Model file for the job. Use its own axes, mm. A direction names the side the tool comes from. Give positions to 0.01 mm unless a question says otherwise; leave off trailing zeros. Write each loop counter-clockwise with the first axis right and the second up, starting at its lowest first coordinate (ties: lowest second). Pieces come first, ordered by that corner, then holes. Notation, with made-up numbers: (-36, 25) - (1, 25) arc R38 cw to (1, 64) - close; hole circle Ø1 at (-24, -14.75). An arc over 180 degrees is marked (long way). Use a Markdown table: item, result. Add a question column.
```python
from build123d import *

# Parameters (mm, degrees)
BOSS_EXTRUDE1_DEPTH = 20
SKETCH8_W           = 42
SKETCH8_H           = 60
CUT_EXTRUDE1_DEPTH  = 15
CUT_EXTRUDE2_START  = -5
CUT_EXTRUDE2_DEPTH  = 5
SKETCH10_R          = 36
CUT_EXTRUDE3_DEPTH  = 159.144630057
SKETCH11_R          = 41
SKETCH11_R_2        = 36
BOSS_EXTRUDE4_DEPTH = 5
SKETCH2_W           = 108.205781707
SKETCH2_H           = 80
SKETCH2_R           = 3
BOSS_EXTRUDE6_DEPTH = 20


# Read off the part's stored shape, not the designer's step: Cut-Extrude2
with BuildPart() as part:
    # Sketch1 → Boss-Extrude1 (new body)
    with BuildSketch(Plane(origin=(0, 0, 0), x_dir=(1, 0, 0), z_dir=(0, 1, 0))):
        with BuildLine():
            Line((47.743715131, 62.553367624), (47.499828545, -45.652139232))
            ThreePointArc((47.499828545, -45.652139232), (-20.152139232, -112.999828545), (-87.499828545, -45.347860768))
            Line((-87.499828545, -45.347860768), (-87.25594196, 62.857646088))
            ThreePointArc((-87.25594196, 62.857646088), (-19.603974182, 130.205335402), (47.743715131, 62.553367624))
        make_face()
    extrude(amount=BOSS_EXTRUDE1_DEPTH)

    # Sketch8 → Cut-Extrude1 (cut)
    with BuildSketch(Plane.XZ):
        with Locations((-20, -62.5)):
            Rectangle(SKETCH8_W, SKETCH8_H)
    extrude(amount=-CUT_EXTRUDE1_DEPTH, mode=Mode.SUBTRACT)

    # Cut-Extrude2 outline → Cut-Extrude2 (cut)
    with BuildSketch(Plane.XZ.offset(-15).offset(CUT_EXTRUDE2_START)):
        with BuildLine():
            Line((-6.5, -34.5), (-6.5, -90.5))
            ThreePointArc((-6.5, -90.5), (-4.5, -92.5), (-2.5, -90.5))
            Line((-2.5, -90.5), (-2.5, -34.5))
            ThreePointArc((-2.5, -34.5), (-4.5, -32.5), (-6.5, -34.5))
        make_face()
        with BuildLine():
            ThreePointArc((-8, -45), (-20, -33), (-32, -45))
            Line((-32, -45), (-32, -80))
            ThreePointArc((-32, -80), (-20, -92), (-8, -80))
            Line((-8, -80), (-8, -45))
        make_face()
        with BuildLine():
            Line((-37.5, -34.5), (-37.5, -90.5))
            ThreePointArc((-37.5, -90.5), (-35.5, -92.5), (-33.5, -90.5))
            Line((-33.5, -90.5), (-33.5, -34.5))
            ThreePointArc((-33.5, -34.5), (-35.5, -32.5), (-37.5, -34.5))
        make_face()
    extrude(amount=CUT_EXTRUDE2_DEPTH, mode=Mode.SUBTRACT)

    # Sketch10 → Cut-Extrude3 (cut, through all)
    with BuildSketch(Plane.XZ):
        with Locations(Location((-20, 45.5, 0), (0, 0, 270))):
            Circle(SKETCH10_R)
    extrude(amount=-CUT_EXTRUDE3_DEPTH, mode=Mode.SUBTRACT)

    # Sketch11 → Boss-Extrude4 (add)
    with BuildSketch(Plane(origin=(0, 20, 0), x_dir=(1, 0, 0), z_dir=(0, 1, 0))):
        with Locations(Location((-20, -45.5, 0), (0, 0, 270))):
            Circle(SKETCH11_R)
        with Locations(Location((-20, -45.5, 0), (0, 0, 90))):
            Circle(SKETCH11_R_2, mode=Mode.SUBTRACT)
    extrude(amount=BOSS_EXTRUDE4_DEPTH)

    # Sketch2 → Boss-Extrude6 (add)
    with BuildSketch(Plane(origin=(47.602482999, 0, 0.107292202), x_dir=(0.002253914548687051, 0, -0.9999974599313777), z_dir=(0.9999974599313777, 0, 0.002253914548687051))):
        with Locations((8.557928136, 40)):
            Rectangle(SKETCH2_W, SKETCH2_H)
        with Locations((-1.551375347, 27.5)):
            Circle(SKETCH2_R, mode=Mode.SUBTRACT)
        with Locations((18.448624653, 27.5)):
            Circle(SKETCH2_R, mode=Mode.SUBTRACT)
        with Locations((18.448624653, 42.5)):
            Circle(SKETCH2_R, mode=Mode.SUBTRACT)
        with Locations((-1.551375347, 42.5)):
            Circle(SKETCH2_R, mode=Mode.SUBTRACT)
    extrude(amount=BOSS_EXTRUDE6_DEPTH)


solid = part.part
```
(1) Band-saw the part on A-A (z = 22). Write the cut outline in (x, y).
(2) Band-saw the part on C-C (y = 56). Write the cut outline in (x, z).
(3) Two-plate mould, pull along X, no slides. Class faces 3 (the cylindrical face through (-21.088, 9.86, -130.192)), 4 (the flat face through (1, 7, -63)): +X half, -X half, draft (parallel to the pull), parting line (faces both ways), or undercut.
(4) Flat gauge pins, fed straight in: pin 1 (3 mm diameter, centred on y = 24.5, z = -48, fed in from +X); pin 2 (4 mm diameter, centred on y = 17, z = -65.5, fed in from +X); pin 3 (7.5 mm diameter, centred on x = -11, y = 7, fed in from +Z). Where does each tip first touch, or does it go through?
(5) Which spindle directions (+Z, -Z, +X, -X, +Y, -Y) get a long thin tool onto all of the face, cutting with end or side? Do faces 1 (the flat face through (-33.5, 18, -63)), 2 (the flat face through (-1, 15, -62)). Say none if no direction does.
(6) Band-saw the part on B-B (x = -20). Write the cut outline in (y, z).
(7) Probe probe 1 along Z at (x, y) = (-20, 7); probe 2 along Z at (x, y) = (-20, 16.75); probe 3 along X at (y, z) = (17.5, 45.5). List the from-to ranges inside material, lowest first. Write a range as [from, to].
(8) Band-saw the part on D-D (z = -27). Write the cut outline in (x, y).
Model answer:
| question | item | result |
|---|---|---|
| 1 | outline | (-87.45, 0) - (-47.27, 0) - (-47.27, 25) - (-53.6, 25) - (-53.6, 20) - (-87.45, 20) - close; (7.27, 0) - (67.55, 0) - (67.55, 80) - (47.55, 80) - (47.55, 20) - (13.6, 20) - (13.6, 25) - (7.27, 25) - close |
| 2 | outline | (47.5, 45.65) - (47.74, -62.55) - (67.74, -62.51) - (67.5, 45.7) - close |
| 3 | face 3 | parting line |
| 3 | face 4 | undercut |
| 4 | pin 1 | stops at x = 67.71 |
| 4 | pin 2 | stops at x = 47.74 |
| 4 | pin 3 | stops at z = 112.8 |
| 5 | face 1 | +Y, -Y |
| 5 | face 2 | -Y |
| 6 | outline | (0, -130.21) - (20, -130.21) - (20, -92) - (15, -92) - (15, -92.5) - (0, -92.5) - close; (0, -32.5) - (15, -32.5) - (15, -33) - (20, -33) - (20, 4.5) - (25, 4.5) - (25, 9.5) - (0, 9.5) - close; (0, 81.5) - (25, 81.5) - (25, 86.5) - (20, 86.5) - (20, 113) - (0, 113) - close |
| 7 | probe 1 | z = [-130.21, -92.5], [-32.5, 9.5], [81.5, 113] |
| 7 | probe 2 | z = [-130.21, -92], [-33, 9.5], [81.5, 113] |
| 7 | probe 3 | x = [-87.5, -56], [16, 67.5] |
| 8 | outline | (-87.34, 0) - (67.66, 0) - (67.66, 80) - (47.66, 80) - (47.66, 20) - (-87.34, 20) - close |
